```python
from build123d import *

# Parameters (mm, degrees)
FASE1_SIZE = 0.2


with BuildPart() as part:
    # Skizze2 → Rotation1 (revolve)
    with BuildSketch(Plane.XY):
        Polygon((3.956451613, 0), (-6.243548387, 0), (-6.243548387, 2), (-5.743548387, 2), (-5.743548387, 1.9), (-5.243548387, 1.9), (-5.243548387, 2), (-1.043548387, 2), (-1.043548387, 3.4), (3.956451613, 3.4), align=None)
    revolve(axis=Axis((3.956451613, 0, 0), (-1, 0, 0)))

    # Fase1
    fase1_edges = [part.edges().sort_by_distance(p)[0] for p in [
        (-6.243548387, -2, 0),
        (3.956451613, -3.4, 0),
    ]]
    chamfer(fase1_edges, length=FASE1_SIZE)


solid = part.part
```
Read the model definition and answer for the solid it produces. Units are mm, in the model's axes. A direction names the side the tool comes from. Coordinates: 2 decimals unless noted, no trailing zeros. Write each loop counter-clockwise with the first axis right and the second up, starting at its lowest first coordinate (ties: lowest second). Pieces come first, ordered by that corner, then holes. Notation, with made-up numbers: (86, 82) -> (114, 82) arc R22 cw to (114, 99) -> close; hole circle Ø11 at (-38.5, 30.25). An arc over 180 degrees is marked (long way). Write item = value, one per line.
(1) Given pin 1 Ø4 at (x, y) = (-2.5, 0.5) entering from +Z; pin 2 Ø1 at (y, z) = (-1, -2.5) entering from -X; pin 3 Ø2 at (x, z) = (-3, -1) entering from +Y, each flat-ended and moving along its own axis, determine where each tip first touches the part or whether it passes through.
From the geometry:
pin_1 = 3.4
pin_2 = -1.04
pin_3 = 2
(2) Section C-C on x = -2 is taken. Write down the section's boundary in (y, z).
From the geometry:
outline = circle Ø4 at (0, 0)
(3) Section D-D on x = 3.25 is taken. Write down the section's boundary in (y, z), plus the area to 3 significant figures.
From the geometry:
outline = circle Ø6.8 at (0, 0)
area = 36.3 mm2
(4) For a pull along X with two mould halves and no side action, classify faces 3 (the face through (-5.49, -1.9, -0.08)), 4 (the face through (-3, 0, 2)), 5 (the face through (3.956, 0, 0)), 6 (the face through (-6.244, 0, 0)) as +X half, -X half, draft (parallel to the pull), parting line (faces both ways), or undercut.
From the geometry:
face_3 = undercut
face_4 = draft
face_5 = +X half
face_6 = -X half
(5) Which of the six approach directions +Z, -Z, +X, -X, +Y, -Y give full straight-line access (tool end or side, diameter ignored) to faces 1 (the face through (-1.044, 0, 2.2)), 2 (the face through (1.39, -0.74, 3.32))?
From the geometry:
face_1 = -X
face_2 = +X, -X
(6) Section A-A on y = 0 is taken. Write down the section's boundary in (x, z), plus the area to 3 significant figures.
From the geometry:
outline = (-6.24, -1.8) -> (-6.04, -2) -> (-5.74, -2) -> (-5.74, -1.9) -> (-5.24, -1.9) -> (-5.24, -2) -> (-1.04, -2) -> (-1.04, -3.4) -> (3.76, -3.4) -> (3.96, -3.2) -> (3.96, 3.2) -> (3.76, 3.4) -> (-1.04, 3.4) -> (-1.04, 2) -> (-5.24, 2) -> (-5.24, 1.9) -> (-5.74, 1.9) -> (-5.74, 2) -> (-6.04, 2) -> (-6.24, 1.8) -> close
area = 54.6 mm2
(7) Straight lines are drawn through the part: L1, parallel to Z at x = -2.25, y = 0; L2, parallel to X at y = -3, z = 0; L3, parallel to Z at x = -0.75, y = 1.25. For each, find the intervals that lie inside material, in ascending order. Write a range as from..to.
From the geometry:
L1 = -2..2
L2 = -1.04..3.96
L3 = -3.16..3.16
